Autodesk Inventor part; units mm, degrees
ref_plane "YZ Plane" through (0, 0, 0) normal (1, 0, 0) x (0, 1, 0)
ref_plane "XZ Plane" through (0, 0, 0) normal (0, 1, 0) x (-1, 0, 0)
ref_plane "XY Plane" through (0, 0, 0) normal (0, 0, 1) x (1, 0, 0)
sketch "Sketch1" plane through (0, 0, 0) normal (0, 1, 0) x (-1, 0, 0)
  line L0 (0, 0) -> (4.8, 0) construction
  line L1 (4.8, 0) -> (4.8, -7.6) construction
  line L2 (4.8, -7.6) -> (0, -7.6) construction
  line L3 (0, -7.6) -> (0, 0) construction
  line L4 (4.8, -9.6) -> (2, -9.6)
  line L5 (2, -9.6) -> (-2, -5.6)
  line L6 (-2, -5.6) -> (-2, -2)
  line L7 (-2, -2) -> (2, 2)
  line L8 (2, 2) -> (4.8, 2)
  line L9 (4.8, 2) -> (4.8, -9.6)
  line L10 (2.4, 0) -> (2.4, 2) construction
  line L11 (-2, -3.8) -> (0, -3.8) construction
  line L12 (2.4, -7.6) -> (2.4, -9.6) construction
  dimension "d0" = 7.6
  dimension "d1" = 4.8
  dimension "d2" = 2
extrude "Extrusion1" add sketch "Sketch1" along normal blind 1.5
sketch "Sketch2" plane through (0, 0, 0) normal (0, -1, 0) x (1, 0, 0)
  line L0 (-4.8, -9.6) -> (-4.8, 2)
  line L1 (0, 0) -> (-4.8, 0)
  line L2 (-4.8, 0) -> (-4.8, -7.6)
  line L3 (-4.8, -7.6) -> (0, -7.6)
  line L4 (0, -7.6) -> (0, 0)
  line L5 (2, -5.6) -> (-2, -9.6)
extrude "Extrusion2" add sketch "Sketch2" along normal blind 7
sketch "Sketch3" plane through (0, 0, 0) normal (1, 0, 0) x (0, 0, -1)
  line L0 (-17.9, 0) -> (-18, 0)
  line L1 (-18, 1) -> (-17.9, 1) construction
  line L2 (0, 0) -> (0, -7)
  line L3 (0, -4) -> (1.7321, -7)
  line L4 (2.8, -7) -> (2.8, 0)
  line L5 (2.8, 0) -> (4.8, 0)
  line L6 (4.8, 0) -> (4.8, -7)
  line L7 (4.8, -7) -> (5.8679, -7)
  line L8 (5.8679, -7) -> (7.6, -4)
  line L9 (7.6, -4) -> (6.3, -4)
  line L10 (6.3, -4) -> (6.3, 0)
  line L11 (7.6, 0) -> (7.6, -7.2498)
  line L12 (6.3, 0) -> (7.6, 0)
  line L13 (2.8, -7) -> (1.7321, -7)
  line L14 (0, -4) -> (1.3, -4)
  line L15 (1.3, -4) -> (1.3, 0)
  line L16 (1.3, 0) -> (0, 0)
  line L17 (0, 0) -> (0, -7)
  line L18 (0, -4) -> (0, -7)
  line L19 (0, -7) -> (1.7321, -7)
  line L20 (7.6, 0) -> (7.6, -4)
  line L21 (3.8, -6.9306) -> (3.8, 0) construction
  line L22 (6.3, -4) -> (4.8, -4) construction
  line L23 (1.3, -4) -> (2.8, -4) construction
  line L24 (-17.9, 0) -> (-18, 0)
  line L25 (-18, 1) -> (-17.9, 1) construction
  line L26 (0, 0) -> (0, -7)
  line L27 (2, 0) -> (5.6, 0)
  line L28 (7.6, -7) -> (0, -7)
  line L29 (2.8, -7) -> (4.8, -7)
  line L30 (5.8679, -7) -> (7.6, -7)
  point P0 (2.8, -7)
  point P1 (4.8, -7)
  dimension "d14" = 4
  dimension "d15" = 1.5
  dimension "d16" = 1
  dimension "d17" = 60
  dimension "d18" = 7.6
  dimension "d20" = 1.3
extrude "Extrusion3" cut sketch "Sketch3" against normal up to surface (4.8 mm away)
fillet "Fillet1" radius 1 2 edges at (-2.4, 0, -4.8) (-2.4, 0, -2.8)
mirror "Mirror1" about plane through (-1.4, 1.5, -3.8) normal (0, 1, 0) of "Extrusion1", "Extrusion2", "Extrusion3", "Fillet1"
properties part number "PlugbothWays"
Work out the finished part from the listing and answer in its coordinate system (mm). A direction names the side the tool comes from. Give positions to 0.01 mm unless a question says otherwise; leave off trailing zeros. Loops run counter-clockwise (first coordinate to the right, second up) from the corner with the lowest first, then second, coordinate; pieces in that order, holes last. Notation, with made-up numbers: M -11.5,58 L 33.5,58 A28 ccw 33.5,80 Z; hole C 47,35.5 d6. An arc over 180 degrees is marked long. One line per item, written item: value. Start each with the question number.
1. Find the intervals of material crossed by probe 1 along Z at (x, y) = (-1.25, 5); probe 2 along Y at (x, z) = (-1.75, -8.25); probe 3 along Z at (x, y) = (-1.5, -5.5), in increasing order.
2. Find section D-D (y = 2). Give the vertices of the cut face in (x, z).
3. Which of the six approach directions +Z, -Z, +X, -X, +Y, -Y give full straight-line access (tool end or side, diameter ignored) to faces 4 (the face through (-2, 7, -1)), 5 (the face through (-2, -4, -2.8)), 6 (the face through (-1, 3, -1))?
4. Each of these flat-tipped pins is pushed along its axis until it touches: P1, Ø2, axis at x = -1.5, y = 4.5, coming from the +Z side; P2, Ø1.4, axis at x = -3, z = -1, coming from the +Y side; P3, Ø1.1, axis at y = -2, z = -6, coming from the +X side. Where does it stop, or does it pass through?
5. Find section A-A (y = 6.25). Give the vertices of the cut face in (x, z).
6. Determine the mould class of faces 1 (the face through (-2, -4, -4.8)), 2 (the face through (-2.366, -5.521, -6.722)), 3 (the face through (2, 2, -4)) for opening direction Z: released by +Z, released by -Z, zero draft, split by the parting line, or undercut.
7. Find section B-B (z = -6.5). Give the vertices of the cut face in (x, y), and give its area (3 significant figures).
Reported:
1. probe 1: z = -6.3 to -4.8, -2.8 to -1.3
1. probe 2: y = 0 to 3
1. probe 3: z = -6.73 to -4.8, -2.8 to -0.87
2. outline: M -4.8,-9.6 L -2,-9.6 L 2,-5.6 L 2,-2 L -2,2 L -4.8,2 Z
3. face 4: +Z, +X, -X
3. face 5: +X, -X, -Y
3. face 6: +X
4. P1: stops at z = -1.3
4. P2: stops at y = 9.94
4. P3: stops at x = 0
5. outline: M -4.8,-6.3 L 0,-6.3 L 0,-4.8 L -4.8,-4.8 Z; M -4.8,-2.8 L 0,-2.8 L 0,-1.3 L -4.8,-1.3 Z
6. face 1: undercut
6. face 2: released by -Z
6. face 3: zero draft
7. outline: M -4.8,-5.91 L 0,-5.91 L 0,-4 L -4.8,-4 Z; M -4.8,0 L 1.1,0 L 1.1,3 L -4.8,3 Z; M -4.8,7 L 0,7 L 0,8.91 L -4.8,8.91 Z
7. area: 36.0 mm²
